```python
from build123d import *

# Parameters (mm, degrees)
RIBCUT1_DEPTH    = 0.428625
RIBCUT2_DEPTH    = 0.6858
RIBCUTSPAT_COUNT = 12
RIBCUTSPAT_ANGLE = 330


with BuildPart() as part:
    # BodySke → BaseBody (revolve)
    with BuildSketch(Plane.XY):
        with BuildLine():
            Line((0, 0), (0, 3.93446))
            Line((0, 3.93446), (0.00508, 3.93446))
            Line((0.00508, 3.93446), (0.00508, 3.93954))
            ThreePointArc((0.00508, 3.93954), (0.34544, 4.2799), (0.6858, 3.93954))
            Line((0.6858, 3.93954), (0.6858, 3.8735))
            Line((0.6858, 3.8735), (1.3716, 3.52425))
            Line((1.3716, 3.52425), (1.3716, 3.175))
            Line((1.3716, 3.175), (18.29435, 3.175))
            Line((18.29435, 3.175), (19.05, 2.41935))
            Line((19.05, 2.41935), (19.05, 0))
            Line((19.05, 0), (0, 0))
        make_face()
    revolve(axis=Axis((0, 0, 0), (1, 0, 0)))

    # RibCut1Ske → RibCut1 (cut)
    with BuildSketch(Plane(origin=(1.3716, 0, 0), x_dir=(0, 0, -1), z_dir=(1, 0, 0))):
        with BuildLine():
            Line((0.41442066, 3.147837435), (0.41442066, 4.259788672))
            ThreePointArc((0.41442066, 4.259788672), (1.107719631, 4.134065944), (1.770995516, 3.896295534))
            Line((1.770995516, 3.896295534), (1.215019898, 2.933317516))
            ThreePointArc((1.215019898, 2.933317516), (0.821750468, 3.066814498), (0.41442066, 3.147837435))
        make_face()
    ribcut1 = extrude(amount=-RIBCUT1_DEPTH, mode=Mode.SUBTRACT)

    # RibCut2Ske → RibCut2 (cut)
    with BuildSketch(Plane(origin=(1.3716, 0, 0), x_dir=(0, 0, -1), z_dir=(1, 0, 0))):
        with BuildLine():
            Line((0.41442066, 3.499799077), (0.41442066, 4.259788672))
            ThreePointArc((0.41442066, 4.259788672), (1.107719631, 4.134065944), (1.770995516, 3.896295534))
            Line((1.770995516, 3.896295534), (1.391000719, 3.238125239))
            ThreePointArc((1.391000719, 3.238125239), (0.91214302, 3.404164093), (0.41442066, 3.499799077))
        make_face()
    ribcut2 = extrude(amount=-RIBCUT2_DEPTH, mode=Mode.SUBTRACT)

    # RibCutsPat: RibCut1, RibCut2 ×12 about axis
    ribcutspat_axis = Axis((0, 0, 0), (1, 0, 0))
    for i in range(1, RIBCUTSPAT_COUNT):
        add(ribcut1.rotate(ribcutspat_axis, i * RIBCUTSPAT_ANGLE / (RIBCUTSPAT_COUNT - 1)), mode=Mode.SUBTRACT)
        add(ribcut2.rotate(ribcutspat_axis, i * RIBCUTSPAT_ANGLE / (RIBCUTSPAT_COUNT - 1)), mode=Mode.SUBTRACT)


solid = part.part
```
Could you check a few things on this model? Use its own coordinates, in mm. A direction names the side the tool comes from. Round coordinates to 2 decimals unless told otherwise and drop trailing zeros. Loops run counter-clockwise (first coordinate to the right, second up) from the corner with the lowest first, then second, coordinate; pieces in that order, holes last. Notation, with made-up numbers: (36.5, 28.5) - (54.5, 28.5) arc R22 ccw to (54.5, 44.5) - close; hole circle Ø11 at (19, 69). An arc over 180 degrees is marked (long way). Answer in a Markdown table with one row per item. Add a question column.
(1) I'm going to push flat-ended pins straight in: pin 1 (4 mm diameter, centred on x = 3, y = -1.5, fed in from -Z); pin 2 (0.8 mm diameter, centred on y = -2, z = 3, fed in from +X); pin 3 (4 mm diameter, centred on y = -3, z = 0.5, fed in from -X); pin 4 (3 mm diameter, centred on x = 4, y = 1, fed in from -Z) (3 decimals). Where does each tip first touch, or does it pass through?
(2) If we section it at C-C (x = 3.75): Please give me the cut outline in (y, z) (3 decimals).
(3) If we mould it in two halves opening along Y, with no side actions, what happens to faces 1 (the face through (0.943, 2.33, -2.4)), 2 (the face through (19.05, 0, 0))? For each: pulls with the +Y half, pulls with the -Y half, needs draft (parallel to the pull), parting line crosses it, or undercut.
(4) I need wall thicknesses on line 1 along Y through (x, z) = (9.25, -1); line 2 along X through (y, z) = (2.5, 3); line 3 along X through (y, z) = (-2.75, 0). Which ranges of each line are inside material? Lowest first, please.
(5) For faces 3 (the face through (0.943, -2.33, 2.4)), 4 (the face through (0, 0, 0)), which set-ups out of +Z, -Z, +X, -X, +Y, -Y let a thin tool reach every point of the face, with its end or its side?
Model answer:
| question | item | result |
|---|---|---|
| 1 | pin 1 | stops at z = -3.53 |
| 1 | pin 2 | stops at x = 1.37 |
| 1 | pin 3 | stops at x = 0 |
| 1 | pin 4 | stops at z = -3.175 |
| 2 | outline | circle Ø6.35 at (0, 0) |
| 3 | face 1 | undercut |
| 3 | face 2 | needs draft |
| 4 | line 1 | y = -3.01 to 3.01 |
| 4 | line 2 | x = 0 to 0.69 |
| 4 | line 3 | x = 0 to 18.72 |
| 5 | face 3 | +X |
| 5 | face 4 | +Z, -Z, -X, +Y, -Y |
